from build123d import *

# Parameters (mm, degrees)
EXTRUDE_1_DEPTH      = 296.2
EXTRUDE_1_DEPTH_BACK = 296.2
CUT_EXTRUDE_1_REACH  = 765.895
SKETCH_3_W           = 20
SKETCH_3_H           = 60
FILLET_1_R           = 100
CUT_EXTRUDE_2_REACH  = 698.157
SKETCH_10_W          = 87
SKETCH_10_H          = 31
SKETCH_11_W          = 20
SKETCH_11_H          = 3
EXTRUDE_2_DEPTH      = 13
SKETCH_12_W          = 20
SKETCH_12_H          = 3
EXTRUDE_3_DEPTH      = 9


with BuildPart() as part:
    # 스케치2 → 보스-돌출1 (new, two sides: drawn at the far end of the back side and taken through both)
    with BuildSketch(Plane(origin=(0, 0, 0), x_dir=(0, 0, -1), z_dir=(1, 0, 0)).offset(-EXTRUDE_1_DEPTH_BACK)):
        with BuildLine():
            Line((-367.271624482, -67.837616249), (-370.190899695, -67.146362149))
            Line((-370.190899695, -67.146362149), (-284.918377839, 292.972961731))
            ThreePointArc((-284.918377839, 292.972961731), (-270.478085605, 315.647309269), (-245.086561619, 324.474459758))
            Line((-245.086561619, 324.474459758), (244.913438381, 324.474459758))
            Line((244.913438381, 324.474459758), (244.913438381, 321.474459758))
            Line((244.913438381, 321.474459758), (-245.086561619, 321.474459758))
            ThreePointArc((-245.086561619, 321.474459758), (-268.617139918, 313.294251439), (-281.999102626, 292.28170763))
            Line((-281.999102626, 292.28170763), (-367.271624482, -67.837616249))
        make_face()
    extrude(amount=EXTRUDE_1_DEPTH + EXTRUDE_1_DEPTH_BACK)

    # 컷-돌출1: up to this plane
    cut_extrude_1_end = Plane(origin=(-296.2, 78.747200123, 332.561859888), z_dir=(0, 0.23041803358111448, 0.9730917376078232))
    # 스케치3 → 컷-돌출1 (cut, up to the surface)
    with BuildSketch(Plane.XY.offset(380), mode=Mode.PRIVATE) as cut_extrude_1_sk1:
        with Locations((-136, -19.036362149)):
            Rectangle(SKETCH_3_W, SKETCH_3_H)
    cut_extrude_1_tool1 = split(extrude(cut_extrude_1_sk1.sketch, amount=-CUT_EXTRUDE_1_REACH, mode=Mode.PRIVATE), bisect_by=cut_extrude_1_end, keep=Keep.BOTH, mode=Mode.PRIVATE)
    add(cut_extrude_1_tool1.solids().sort_by_distance((-136, -19.036362, 380))[0], mode=Mode.SUBTRACT)
    # 스케치3 → 컷-돌출1 (cut, up to the surface)
    with BuildSketch(Plane.XY.offset(380), mode=Mode.PRIVATE) as cut_extrude_1_sk2:
        with Locations((136, -19.036362149)):
            Rectangle(SKETCH_3_W, SKETCH_3_H)
    cut_extrude_1_tool2 = split(extrude(cut_extrude_1_sk2.sketch, amount=-CUT_EXTRUDE_1_REACH, mode=Mode.PRIVATE), bisect_by=cut_extrude_1_end, keep=Keep.BOTH, mode=Mode.PRIVATE)
    add(cut_extrude_1_tool2.solids().sort_by_distance((136, -19.036362, 380))[0], mode=Mode.SUBTRACT)

    # 필렛1
    fillet_1_edges = [part.edges().sort_by_distance(p)[0] for p in [
        (296.2, -67.491989199, 368.731262089),
        (-296.2, -67.491989199, 368.731262089),
    ]]
    fillet(fillet_1_edges, radius=FILLET_1_R)

    # 스케치10 → 컷-돌출2 (cut, up to next)
    with BuildSketch(Plane(origin=(0, 79.438454224, 335.4811351), x_dir=(1, 0, 0), z_dir=(0, 0.23041803358111446, 0.9730917376078232)), mode=Mode.PRIVATE) as cut_extrude_2_sk1:
        with Locations((0, 183.93923605)):
            Rectangle(SKETCH_10_W, SKETCH_10_H)
    cut_extrude_2_tool1 = extrude(cut_extrude_2_sk1.sketch, amount=-CUT_EXTRUDE_2_REACH, mode=Mode.PRIVATE) & part.part
    add(cut_extrude_2_tool1.solids().sort_by_distance((0, 258.428205, 293.098218))[0], mode=Mode.SUBTRACT)

    # 스케치11 → 보스-돌출2 (add)
    with BuildSketch(Plane(origin=(0, 79.438454224, 335.4811351), x_dir=(1, 0, 0), z_dir=(0, 0.23041803358111446, 0.9730917376078232))):
        with Locations((251.9, -106.338229375)):
            Rectangle(SKETCH_11_W, SKETCH_11_H)
    extrude_2 = extrude(amount=-EXTRUDE_2_DEPTH)

    # 스케치12 → 보스-돌출3 (add)
    with BuildSketch(Plane(origin=(0, -102.01721479, 24.156618657), x_dir=(1, 0, 0), z_dir=(0, 0.9730917376078232, -0.23041803358111443))):
        with Locations((251.9, -333.257973102)):
            Rectangle(SKETCH_12_W, SKETCH_12_H)
    extrude_3 = extrude(amount=EXTRUDE_3_DEPTH)

    # 대칭 복사1: 보스-돌출2, 보스-돌출3 across plane
    add(extrude_2.mirror(Plane(origin=(0, 0, 0), x_dir=(0, 0, 1), z_dir=(1, 0, 0))))
    add(extrude_3.mirror(Plane(origin=(0, 0, 0), x_dir=(0, 0, 1), z_dir=(1, 0, 0))))


solid = part.part
Design review of the part built by this model. Coordinates are the model's own, in mm. Give positions to 0.01 mm unless a question says otherwise; leave off trailing zeros. Write each loop counter-clockwise with the first axis right and the second up, starting at its lowest first coordinate (ties: lowest second). Pieces come first, ordered by that corner, then holes. Notation, with made-up numbers: M -40,24 L -6,24 A32 cw -6,52 Z; hole C -17,69 d8. An arc over 180 degrees is marked long. Return JSON: item names as keys, results as strings. Group by question number.
Item 1: Take a section at D-D (y = 152). Give the boundary of the cut face in (x, z), plus the area to 3 significant figures.
Item 2: Take a section at C-C (z = 91). Give the boundary of the cut face in (x, y), plus the area to 3 significant figures.
Item 3: Wall thickness on line 1 along Y through (x, z) = (-171.5, 179.5); line 2 along Y through (x, z) = (56, 247); line 3 along Z through (x, y) = (25, 185): over which ranges is each line inside the solid? List them lowest first.
Item 4: Take a section at B-B (x = 86.5). Give the boundary of the cut face in (y, z).
Item 5: Take a section at A-A (x = -8). Give the boundary of the cut face in (y, z).
Item 6: Clearance check with flat-ended pins moving along their axes: pin 1 Ø10 at (y, z) = (-21.5, 351) entering from +X; pin 2 Ø5 at (x, y) = (-118, 111) entering from +Z; pin 3 Ø5 at (y, z) = (-29.5, 356) entering from -X. State where each tip first meets the part, or that it passes through.
Item 7: The part is to be moulded in two halves that separate along X. For faces 1 (the flat face through (126, -19, 357)), 2 (the cylindrical face through (266.13, -39.74, 362.18)), 3 (the flat face through (-4, 321.474, -3)), say which applies: pulls with the +X half, pulls with the -X half, needs draft (parallel to the pull), parting line crosses it, or undercut.
Return value:
{
 "1": {"outline": "M -296.2,315.22 L 296.2,315.22 L 296.2,318.3 L -296.2,318.3 Z", "area": "1,830 mm2"},
 "2": {"outline": "M -296.2,321.47 L 296.2,321.47 L 296.2,324.47 L -296.2,324.47 Z", "area": "1,780 mm2"},
 "3": {"line 1": "y = 321.47 to 324.47", "line 2": "y = 321.43 to 324.43", "line 3": "z = 307.4 to 310.49"},
 "4": {"outline": "M -67.84,367.27 L 292.28,282 A37.93 cw 321.47,245.09 L 321.47,-244.91 L 324.47,-244.91 L 324.47,245.09 A40.93 ccw 292.97,284.92 L -67.15,370.19 Z"},
 "5": {"outline": "M -67.84,367.27 L 242.65,293.75 L 243.35,296.67 L -67.15,370.19 Z; M 272.82,286.61 L 292.28,282 A37.93 cw 321.47,245.09 L 321.47,-244.91 L 324.47,-244.91 L 324.47,245.09 A40.93 ccw 292.97,284.92 L 273.51,289.53 Z"},
 "6": {"pin 1": "stops at x = 261.9", "pin 2": "stops at z = 328.6", "pin 3": "stops at x = -277.09"},
 "7": {"face 1": "undercut", "face 2": "pulls with the +X half", "face 3": "needs draft"}
}
